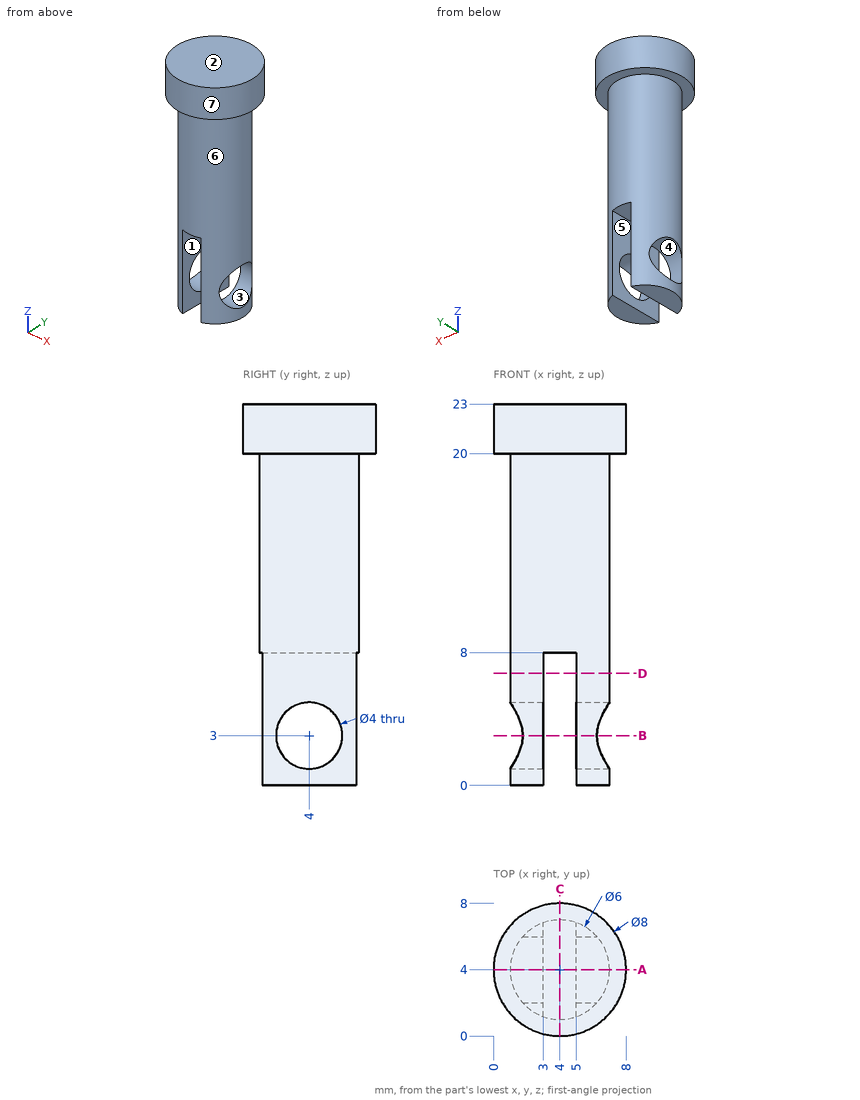
The drawing under review shows one solid part. Ordinate dimensions are in mm from its lowest x, y, z. A direction names the side the tool comes from. Give positions to 0.01 mm unless a question says otherwise; leave off trailing zeros. Order: outer loops, then holes, each group sorted by start corner. A loop starts at its lowest first (then second) coordinate and runs counter-clockwise, first axis right, second up. Notation, with made-up numbers: M 19,31.25 L 62,31.25 A11 ccw 62,46.25 Z; hole C -35,-26 d9. An arc over 180 degrees is marked long. Answer in a Markdown table with one row per item. Add a question column.
1. Add section C-C on x = 4. State the section outline as (y, z) points, plus the area to 3 significant figures.
2. For pin 1 Ø1.7 at (y, z) = (4.5, 5.5) entering from +X; pin 2 Ø3 at (y, z) = (2.5, 2) entering from -X; pin 3 Ø1 at (x, z) = (6.5, 8.5) entering from +Y, all flat-tipped, find the tip position at first contact; note any pin that passes through.
3. Machinability: for the marked faces 5, 6 and 7, which of the approach directions +Z, -Z, +X, -X, +Y, -Y give a long, thin tool a straight path to every point of the face, cutting with its end or side? Answer none if there is none.
4. Add section B-B on z = 3. State the section outline as (x, y) points.
5. To check wall thickness, follow line 1 along Z through (x, y) = (2.1, 4); line 2 along Z through (x, y) = (3.25, 5); line 3 along Y through (x, z) = (6.25, 1.75). State the ranges of each line that lie inside material, in increasing order.
6. Add section A-A on y = 4. State the section outline as (x, z) points, plus the area to 3 significant figures.
7. Mouldability with a two-part tool opening along Z and no side actions: class the marked faces 1, 2, 3 and 4 as released by +Z, released by -Z, zero draft, split by the parting line, or undercut.
8. Add section D-D on z = 6.75. State the section outline as (x, y) points.
The answers:
| question | item | result |
|---|---|---|
| 1 | outline | M 0,20 L 1,20 L 1,8 L 7,8 L 7,20 L 8,20 L 8,23 L 0,23 Z |
| 1 | area | 96.0 mm2 |
| 2 | pin 1 | x = 7 |
| 2 | pin 2 | x = 1.02 |
| 2 | pin 3 | y = 6.24 |
| 3 | face 5 | -Z, +Y, -Y |
| 3 | face 6 | -Z |
| 3 | face 7 | +Z, -Z |
| 4 | outline | M 1.76,2 A3 ccw 3,1.17 L 3,2 Z; M 1.76,6 L 3,6 L 3,6.83 A3 ccw Z; M 5,1.17 A3 ccw 6.24,2 L 5,2 Z; M 5,6 L 6.24,6 A3 ccw 5,6.83 Z |
| 5 | line 1 | 0 to 1, 5 to 23 |
| 5 | line 2 | 8 to 23 |
| 5 | line 3 | 2.02 to 2.44, 5.56 to 5.98 |
| 6 | outline | M 0,20 L 1,20 L 1,5 L 3,5 L 3,8 L 5,8 L 5,5 L 7,5 L 7,20 L 8,20 L 8,23 L 0,23 Z; M 1,0 L 3,0 L 3,1 L 1,1 Z; M 5,0 L 7,0 L 7,1 L 5,1 Z |
| 6 | area | 112 mm2 |
| 7 | face 1 | zero draft |
| 7 | face 2 | released by +Z |
| 7 | face 3 | undercut |
| 7 | face 4 | undercut |
| 8 | outline | M 3,1.17 L 3,6.83 A3 ccw Z; M 5,1.17 A3 ccw 5,6.83 Z |
